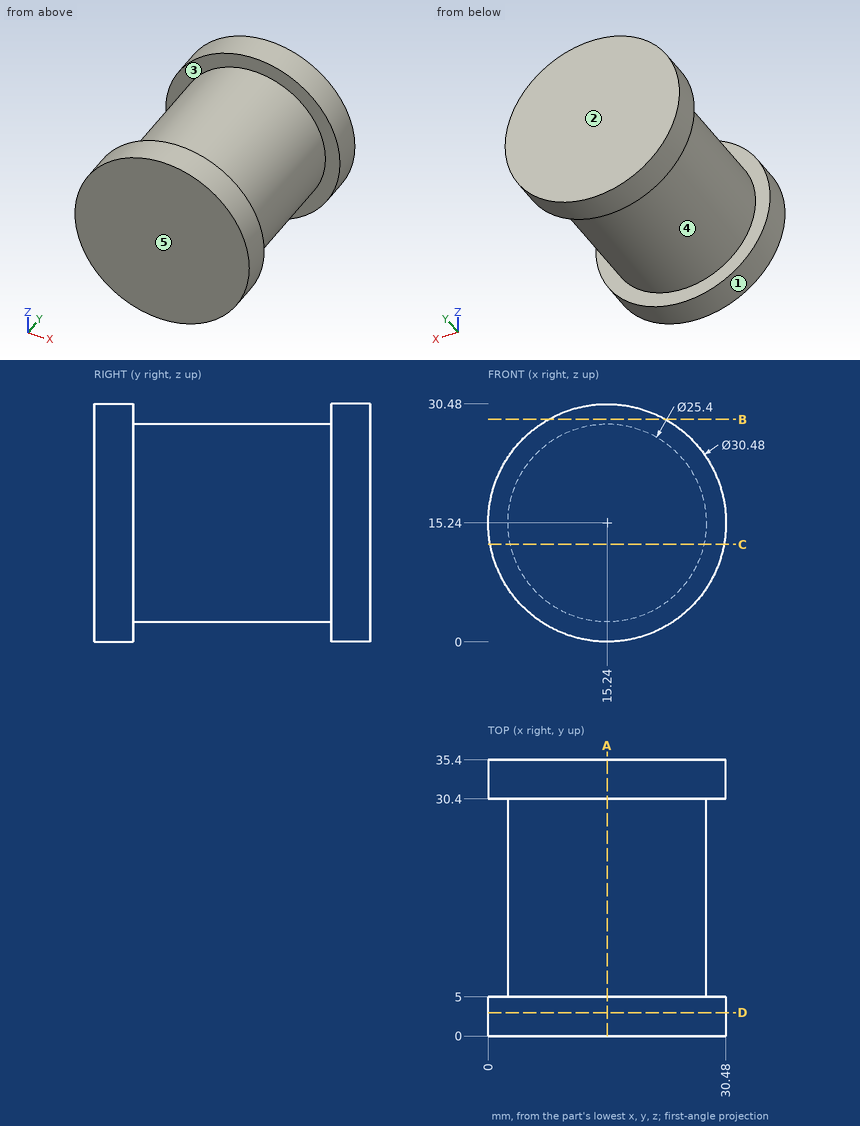
The drawing under review shows one solid part. Ordinate dimensions are in mm from its lowest x, y, z. A direction names the side the tool comes from. Coordinates: 2 decimals unless noted, no trailing zeros. Order: outer loops, then holes, each group sorted by start corner. A loop starts at its lowest first (then second) coordinate and runs counter-clockwise, first axis right, second up. Notation, with made-up numbers: (-26, 54) -> (-11, 54) arc R18 ccw to (-11, 70) -> close; hole circle Ø10 at (-32.5, 41.5). An arc over 180 degrees is marked (long way). Answer in a Markdown table with one row per item.
(1) Consider section D-D (y = 3). Write out the cut boundary in (x, z), plus the area to 3 significant figures.
Answers:
| item | result |
|---|---|
| outline | circle Ø30.48 at (15.24, 15.24) |
| area | 730 mm² |
(2) Insertion check: pin 1 (3 mm diameter, centred on y = 30, z = 4.5, fed in from -X); pin 2 (4 mm diameter, centred on y = 4.5, z = 23.5, fed in from +X); pin 3 (4 mm diameter, centred on x = 6.5, y = 31.5, fed in from -Z). Each pin has a flat end and moves straight along its axis. Give the tip position at first contact, or say it passes through.
Answers:
| item | result |
|---|---|
| pin 1 | x = 3.16 |
| pin 2 | x = 29.13 |
| pin 3 | z = 1.57 |
(3) Consider section A-A (x = 15.24). Write out the cut boundary in (y, z).
Answers:
| item | result |
|---|---|
| outline | (0, 0) -> (5, 0) -> (5, 2.54) -> (30.4, 2.54) -> (30.4, 0) -> (35.4, 0) -> (35.4, 30.48) -> (30.4, 30.48) -> (30.4, 27.94) -> (5, 27.94) -> (5, 30.48) -> (0, 30.48) -> close |
(4) Wall thickness on line 1 along Y through (x, z) = (9.5, 27.5); line 2 along X through (y, z) = (31, 15); line 3 along Z through (x, y) = (6.5, 3): over which ranges is each line inside the solid? List them lowest first.
Answers:
| item | result |
|---|---|
| line 1 | 0 to 5, 30.4 to 35.4 |
| line 2 | 0 to 30.48 |
| line 3 | 2.76 to 27.72 |
(5) The part is to be moulded in two halves that separate along Y. For the marked faces 1, 2 and 3, say which applies: +Y half, -Y half, draft (parallel to the pull), parting line (faces both ways), or undercut.
Answers:
| item | result |
|---|---|
| face 1 | draft |
| face 2 | +Y half |
| face 3 | undercut |
(6) Machinability: for the marked faces 4 and 5, which of the approach directions +Z, -Z, +X, -X, +Y, -Y give a long, thin tool a straight path to every point of the face, cutting with its end or side? Answer none if there is none.
Answers:
| item | result |
|---|---|
| face 4 | none |
| face 5 | +Z, -Z, +X, -X, -Y |
(7) Consider section B-B (z = 28.5). Write out the cut boundary in (x, y).
Answers:
| item | result |
|---|---|
| outline | (7.73, 0) -> (22.75, 0) -> (22.75, 5) -> (7.73, 5) -> close; (7.73, 30.4) -> (22.75, 30.4) -> (22.75, 35.4) -> (7.73, 35.4) -> close |
(8) Consider section C-C (z = 12.5). Write out the cut boundary in (x, y).
Answers:
| item | result |
|---|---|
| outline | (0.25, 0) -> (30.23, 0) -> (30.23, 5) -> (27.64, 5) -> (27.64, 30.4) -> (30.23, 30.4) -> (30.23, 35.4) -> (0.25, 35.4) -> (0.25, 30.4) -> (2.84, 30.4) -> (2.84, 5) -> (0.25, 5) -> close |
